CAD build for the part. Positions are in the model's coordinates, mm. Face numbers are marked on the shaded views. A direction names the side the tool comes from. Coordinates: 2 decimals unless noted, no trailing zeros. Write each loop counter-clockwise with the first axis right and the second up, starting at its lowest first coordinate (ties: lowest second). Pieces come first, ordered by that corner, then holes. Notation, with made-up numbers: M 32,-29 L 45,-29 A5 ccw 45,-25 Z; hole C -38.5,53.25 d9. An arc over 180 degrees is marked long. Put each result on its own line as item: value. Start each with the question number.
```python
from build123d import *

# Parameters (mm, degrees)
F1_DEPTH = 101.6
F2_R     = 50.79999
F3_R     = 31.75
F4_DEPTH = 38.1


# Not quite as in the source:
# - a fillet or chamfer is up to 0.001 mm smaller than in the source, because OpenCascade refuses the exact size
# - the program builds the solid bodies; features that only make, move or delete a surface that nothing else refers to are left out


with BuildPart() as f1:
    # F0 (on Front) → F1 (new body)
    with BuildSketch(Plane.XZ):
        Polygon((-74.6155765653, -32.5891098499), (-74.6155765653, -51.6391098499), (84.1344234347, -51.6391098499), (84.1344234347, -79.0963023901), (84.1344234347, -83.3891098499), (103.1844234347, -83.3891098499), (103.1844234347, -32.5891098499), align=None)
    extrude(amount=F1_DEPTH)

    # F2 (radius 50.8 in the source; OpenCascade refuses exactly that, so slightly less here)
    f2_edges = [f1.edges().sort_by_distance(p)[0] for p in [
        (-74.615577, 0, -42.11411),
        (-74.615577, -101.6, -42.11411),
    ]]
    fillet(f2_edges, radius=F2_R)

    # F3 (on face) → F4 (join)
    with BuildSketch(Plane.XY.offset(-32.5891098499)):
        with Locations((-23.8155765653, -50.8)):
            Circle(F3_R)
    extrude(amount=F4_DEPTH)


solid = f1.part
```
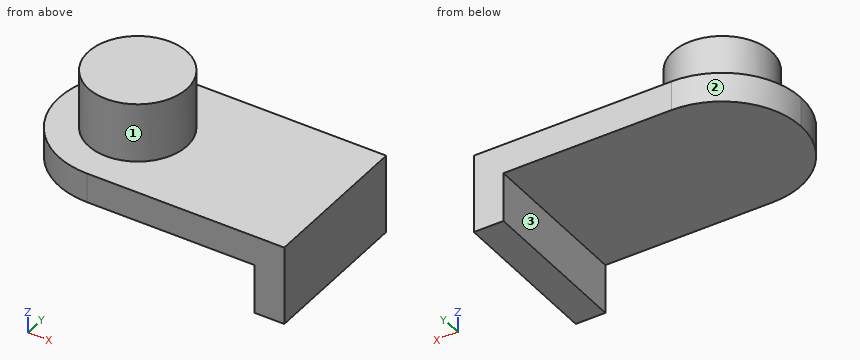
(1) Slice it at B-B, the plane x = 17. Write the cut outline in (y, z), then the cut area to 3 significant figures.
(2) Drop flat-ended pins along their axis: pin 1 (10 mm diameter, centred on y = -64.5, z = -21, fed in from -X); pin 2 (1 mm diameter, centred on y = -25, z = -7, fed in from +X); pin 3 (3 mm diameter, centred on x = -54, z = -25.5, fed in from +Y). Give the stop position or say it passes through.
(3) Drill centre lines: line 1 (X direction, y = -12, z = -76.5); line 2 (Z direction, x = 94, y = -65); line 3 (Z direction, x = 0, y = -44.5). Where is each one in solid material? Low to high. Write a range as [from, to].
(4) Slice it at A-A, the plane z = -16.5. Write the cut outline in (x, y), then the cut area to 3 significant figures.
(5) Which spindle directions (+Z, -Z, +X, -X, +Y, -Y) get a long thin tool onto all of the face, cutting with end or side? Do the marked faces 1, 2 and 3. Say none if no direction does.
(6) Slice it at C-C, the plane y = -93. Write the cut outline in (x, z).
(7) Slice it at D-D, the plane y = -7.5. Write the cut outline in (x, z).
Result set:
1. outline: M -101.6,-51.64 L 0,-51.64 L 0,-32.59 L -101.6,-32.59 Z
1. area: 1,940 mm^2
2. pin 1: stops at x = -54.35
2. pin 2: stops at x = -4.63
2. pin 3: stops at y = -37.19
3. line 1: x = [84.13, 103.18]
3. line 2: z = [-83.39, -32.59]
3. line 3: z = [-51.64, 5.51]
4. outline: C -23.82,-50.8 d63.5
4. area: 3,170 mm^2
5. face 1: +Z
5. face 2: +Z, -Z, -X, +Y
5. face 3: -Z, -X, +Y, -Y
6. outline: M -52.1,-51.64 L 84.13,-51.64 L 84.13,-83.39 L 103.18,-83.39 L 103.18,-32.59 L -52.1,-32.59 Z
7. outline: M -50.38,-51.64 L 84.13,-51.64 L 84.13,-83.39 L 103.18,-83.39 L 103.18,-32.59 L -50.38,-32.59 Z
